Geometry: final body of the model. Coordinates: model frame, mm. Face numbers are marked on the shaded views. Round coordinates to 2 decimals unless told otherwise and drop trailing zeros. Loops run counter-clockwise (first coordinate to the right, second up) from the corner with the lowest first, then second, coordinate; pieces in that order, holes last. Notation, with made-up numbers: (72, -22.5) - (119, -22.5) arc R5 ccw to (119, -14.5) - close; hole circle Ø1 at (85.25, 61.5). An arc over 180 degrees is marked (long way). Return JSON: item names as keys, results as strings. Group by question number.
1. Section B-B on y = 0. Return loops of the section in (x, z), and give its area (3 significant figures).
2. Section C-C on z = -18. Return loops of the section in (x, y).
3. Draft query along Y for the marked faces 1, 2, 3 and 4. Return one class per face: +Y half, -Y half, draft (parallel to the pull), parting line (faces both ways), or undercut.
4. First-contact query: pin 1 Ø11.5 at (x, y) = (245.36, -30.16) entering from +Z; pin 2 Ø25 at (x, y) = (245.36, 30.16) entering from -Z. Flat tips, straight axial feed; report the tip coordinate or a pass-through.
5. Section A-A on x = 0. Return loops of the section in (y, z).
6. Section D-D on y = -35. Return loops of the section in (x, z), and give its area (3 significant figures).
7. Material intervals for probe 1 along Y at (x, z) = (0, 41); probe 2 along Z at (x, y) = (228, 11.5); probe 3 along Y at (x, z) = (-243, -16.5), sorted ascending.
from build123d import *

# Parameters (mm, degrees)
BOSS_EXTRUDE1_DEPTH = 279.4
CUT_EXTRUDE1_REACH  = 78.2
SKETCH2_R           = 25.4
CUT_EXTRUDE2_REACH  = 78.2
SKETCH3_R           = 9.525


with BuildPart() as part:
    # Sketch1 → Boss-Extrude1 (new body, symmetric)
    with BuildSketch(Plane(origin=(0, 0, 0), x_dir=(0, 0, -1), z_dir=(1, 0, 0))):
        with BuildLine():
            Line((-48.8061, -76.2), (-48.8061, 76.2))
            Line((-48.8061, 76.2), (27.3939, 76.2))
            Line((27.3939, 76.2), (27.3939, 73.710744653))
            ThreePointArc((27.3939, 73.710744653), (26.604945151, 71.66452399), (24.646512202, 70.677604975))
            Line((24.646512202, 70.677604975), (-32.895230506, 64.974685943))
            ThreePointArc((-32.895230506, 64.974685943), (-37.791312879, 62.507388407), (-39.7637, 57.391836749))
            Line((-39.7637, 57.391836749), (-39.7637, -57.391836749))
            ThreePointArc((-39.7637, -57.391836749), (-37.791312879, -62.507388407), (-32.895230506, -64.974685943))
            Line((-32.895230506, -64.974685943), (24.646512202, -70.677604975))
            ThreePointArc((24.646512202, -70.677604975), (26.604945151, -71.66452399), (27.3939, -73.710744653))
            Line((27.3939, -73.710744653), (27.3939, -76.2))
            Line((27.3939, -76.2), (-48.8061, -76.2))
        make_face()
    extrude(amount=BOSS_EXTRUDE1_DEPTH, both=True)

    # Sketch2 → Cut-Extrude1 (cut, up to next)
    with BuildSketch(Plane.XY.offset(48.8061), mode=Mode.PRIVATE) as cut_extrude1_sk1:
        Circle(SKETCH2_R)
    cut_extrude1_tool1 = extrude(cut_extrude1_sk1.sketch, amount=-CUT_EXTRUDE1_REACH, mode=Mode.PRIVATE) & part.part
    add(cut_extrude1_tool1.solids().sort_by_distance((0, 0, 48.8061))[0], mode=Mode.SUBTRACT)

    # Sketch3 → Cut-Extrude2 (cut, up to next)
    with BuildSketch(Plane.XY.offset(48.8061), mode=Mode.PRIVATE) as cut_extrude2_sk1:
        with Locations((-245.364, 30.1625)):
            Circle(SKETCH3_R)
    cut_extrude2_tool1 = extrude(cut_extrude2_sk1.sketch, amount=-CUT_EXTRUDE2_REACH, mode=Mode.PRIVATE) & part.part
    add(cut_extrude2_tool1.solids().sort_by_distance((-245.364, 30.1625, 48.8061))[0], mode=Mode.SUBTRACT)
    # Sketch3 → Cut-Extrude2 (cut, up to next)
    with BuildSketch(Plane.XY.offset(48.8061), mode=Mode.PRIVATE) as cut_extrude2_sk2:
        with Locations((245.364, 30.1625)):
            Circle(SKETCH3_R)
    cut_extrude2_tool2 = extrude(cut_extrude2_sk2.sketch, amount=-CUT_EXTRUDE2_REACH, mode=Mode.PRIVATE) & part.part
    add(cut_extrude2_tool2.solids().sort_by_distance((245.364, 30.1625, 48.8061))[0], mode=Mode.SUBTRACT)
    # Sketch3 → Cut-Extrude2 (cut, up to next)
    with BuildSketch(Plane.XY.offset(48.8061), mode=Mode.PRIVATE) as cut_extrude2_sk3:
        with Locations((245.364, -30.1625)):
            Circle(SKETCH3_R)
    cut_extrude2_tool3 = extrude(cut_extrude2_sk3.sketch, amount=-CUT_EXTRUDE2_REACH, mode=Mode.PRIVATE) & part.part
    add(cut_extrude2_tool3.solids().sort_by_distance((245.364, -30.1625, 48.8061))[0], mode=Mode.SUBTRACT)
    # Sketch3 → Cut-Extrude2 (cut, up to next)
    with BuildSketch(Plane.XY.offset(48.8061), mode=Mode.PRIVATE) as cut_extrude2_sk4:
        with Locations((-245.364, -30.1625)):
            Circle(SKETCH3_R)
    cut_extrude2_tool4 = extrude(cut_extrude2_sk4.sketch, amount=-CUT_EXTRUDE2_REACH, mode=Mode.PRIVATE) & part.part
    add(cut_extrude2_tool4.solids().sort_by_distance((-245.364, -30.1625, 48.8061))[0], mode=Mode.SUBTRACT)


solid = part.part
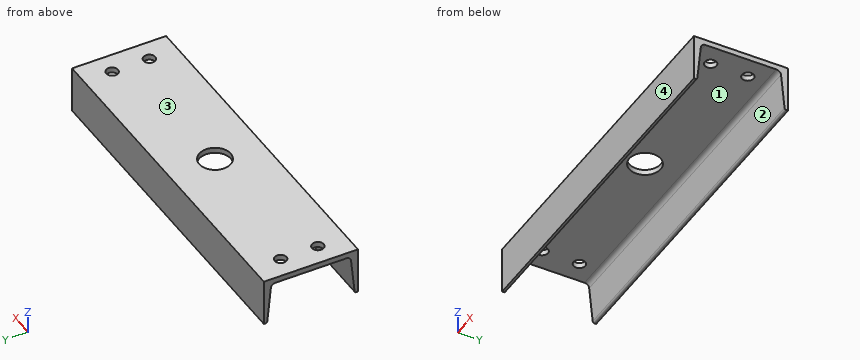
Taken from the geometry:
{
 "1": {"outline": "(-279.4, 39.76) - (-25.4, 39.76) - (-25.4, 48.81) - (-279.4, 48.81) - close; (25.4, 39.76) - (279.4, 39.76) - (279.4, 48.81) - (25.4, 48.81) - close", "area": "4,590 mm2"},
 "2": {"outline": "(-279.4, -76.2) - (279.4, -76.2) - (279.4, -70.02) - (-279.4, -70.02) - close; (-279.4, 70.02) - (279.4, 70.02) - (279.4, 76.2) - (-279.4, 76.2) - close"},
 "3": {"face 1": "undercut", "face 2": "undercut", "face 3": "draft", "face 4": "-Y half"},
 "4": {"pin 1": "through", "pin 2": "z = 39.76"},
 "5": {"outline": "(-76.2, -27.39) - (-73.71, -27.39) arc R3.05 ccw to (-70.68, -24.65) - (-64.97, 32.9) arc R7.62 cw to (-57.39, 39.76) - (-25.4, 39.76) - (-25.4, 48.81) - (-76.2, 48.81) - close; (25.4, 39.76) - (57.39, 39.76) arc R7.62 cw to (64.97, 32.9) - (70.68, -24.65) arc R3.05 ccw to (73.71, -27.39) - (76.2, -27.39) - (76.2, 48.81) - (25.4, 48.81) - close"},
 "6": {"outline": "(-279.4, 39.76) - (-253.57, 39.76) - (-253.57, 48.81) - (-279.4, 48.81) - close; (-237.16, 39.76) - (237.16, 39.76) - (237.16, 48.81) - (-237.16, 48.81) - close; (253.57, 39.76) - (279.4, 39.76) - (279.4, 48.81) - (253.57, 48.81) - close", "area": "4,760 mm2"},
 "7": {"probe 1": "-76.2 to -25.4, 25.4 to 76.2", "probe 2": "39.76 to 48.81", "probe 3": "-76.2 to -69.87, 69.87 to 76.2"}
}
